from build123d import *

# Parameters (mm, degrees)
SKETCH_2_R          = 2.5
EXTRUDE_1_DEPTH     = 50
CUT_EXTRUDE_START   = -15
CUT_EXTRUDE_1_DEPTH = 20
SKETCH_5_W          = 20
SKETCH_5_H          = 15
EXTRUDE_2_DEPTH     = 2.5


with BuildPart() as part:
    # 草图2 → 凸台-拉伸1 (new body)
    with BuildSketch(Plane(origin=(0, 0, 0), x_dir=(0, 0, -1), z_dir=(1, 0, 0))):
        Circle(SKETCH_2_R)
    extrude(amount=-EXTRUDE_1_DEPTH)

    # 草图4 → 切除-拉伸1 (cut)
    with BuildSketch(Plane(origin=(0, 0, 0), x_dir=(0, 0, -1), z_dir=(1, 0, 0)).offset(CUT_EXTRUDE_START)):
        with BuildLine():
            Line((-2.5, 0), (2.5, 0))
            ThreePointArc((2.5, 0), (0, 2.5), (-2.5, 0))
        make_face()
    extrude(amount=-CUT_EXTRUDE_1_DEPTH, mode=Mode.SUBTRACT)

    # 草图5 → 凸台-拉伸2 (add)
    with BuildSketch(Plane(origin=(0, 0, 0), x_dir=(1, 0, 0), z_dir=(0, 1, 0))):
        with Locations((-25, 0)):
            Rectangle(SKETCH_5_W, SKETCH_5_H)
    extrude(amount=EXTRUDE_2_DEPTH)


solid = part.part
Verification items for the finished model (mm, model axes). A direction names the side the tool comes from. Round coordinates to 2 decimals unless told otherwise and drop trailing zeros. Write each loop counter-clockwise with the first axis right and the second up, starting at its lowest first coordinate (ties: lowest second). Pieces come first, ordered by that corner, then holes.
(1) Access from +Z, -Z, +X, -X, +Y, -Y to the whole of each face (thin tool, end or side, straight path). Record for faces 1 (the flat face through (-25, 0, 5)), 2 (the flat face through (-25, 0, -5)), 3 (the cylindrical face through (-24.65, -2.44, 0.54)), 4 (the flat face through (-25, 2.5, 0)), 5 (the flat face through (0, 0, 0)).
Returned:
face 1: +Z, +X, -X, -Y
face 2: -Z, +X, -X, -Y
face 3: none
face 4: +Z, -Z, +X, -X, +Y
face 5: +Z, -Z, +X, +Y, -Y
(2) Material ranges on line 1 (X direction, y = 0.4, z = 6.75); line 2 (Y direction, x = -30.5, z = -4.25); line 3 (Y direction, x = -6.5, z = 0.25), recorded low to high.
Returned:
line 1: x = -35 to -15
line 2: y = 0 to 2.5
line 3: y = -2.49 to 2.49
(3) Section check B-B (y = 1.7). Enter the section's corners in (x, z).
Returned:
outline: (-50, -1.83) - (-35, -1.83) - (-35, -7.5) - (-15, -7.5) - (-15, -1.83) - (0, -1.83) - (0, 1.83) - (-15, 1.83) - (-15, 7.5) - (-35, 7.5) - (-35, 1.83) - (-50, 1.83) - close
(4) Section check C-C (z = 4.5). Enter the section's corners in (x, y).
Returned:
outline: (-35, 0) - (-15, 0) - (-15, 2.5) - (-35, 2.5) - close
(5) Depth check by flat-ended pin: pin 1 Ø2 at (y, z) = (1, 5) entering from -X; pin 2 Ø1.2 at (y, z) = (1.5, -3) entering from +X; pin 3 Ø1.5 at (x, z) = (-21.5, 4.5) entering from -Y. Enter the tip coordinate at first touch or a pass-through.
Returned:
pin 1: stops at x = -35
pin 2: stops at x = -15
pin 3: stops at y = 0
(6) Section check A-A (x = -34). Enter the section's corners in (y, z).
Returned:
outline: (0, -7.5) - (2.5, -7.5) - (2.5, 7.5) - (0, 7.5) - (0, 2.5) arc R2.5 ccw to (0, -2.5) - close
(7) Section check D-D (x = -5). Enter the section's corners in (y, z), plus the area to 3 significant figures.
Returned:
outline: circle Ø5 at (0, 0)
area: 19.6 mm2
